Geometry: final body of the model. Coordinates: model frame, mm. Face numbers are marked on the shaded views. A direction names the side the tool comes from. Coordinates: 2 decimals unless noted, no trailing zeros. Order: outer loops, then holes, each group sorted by start corner. A loop starts at its lowest first (then second) coordinate and runs counter-clockwise, first axis right, second up. Notation, with made-up numbers: M 18.25,-35.75 L 35.25,-35.75 A15 ccw 35.25,-9.75 Z; hole C 79,-8 d7. An arc over 180 degrees is marked long. Use CSV: the item, a comma, the result in double quotes. Start each with the question number.
Q1. Mould query, pull axis Y, two halves, no side actions, for the marked faces 1, 2 and 3. Classes: +Y half, -Y half, draft (parallel to the pull), parting line (faces both ways), or undercut.
Q2. Section query C-C, the plane x = 0. Output: boundary loops of the cut face in (y, z).
Q3. Section query B-B, the plane y = 0. Output: boundary loops of the cut face in (x, z), and give its area (3 significant figures).
Q4. Section query A-A, the plane x = 8. Output: boundary loops of the cut face in (y, z), and give its area (3 significant figures).
Q5. Ray query, probe 1 along Y at (x, z) = (8, 1.35); probe 2 along Y at (x, z) = (4.5, 6.75); probe 3 along X at (y, z) = (0.25, 2). Return the intervals inside material, ascending.
Q6. Section query D-D, the plane z = 11.5. Output: boundary loops of the cut face in (x, y).
Q7. Access query for the marked faces 4, 5, 6, 7 and 8. Directions: +Z, -Z, +X, -X, +Y, -Y. A direction counts if a zero-diameter tool reaches every point of the face in a straight line with its end or side. Return the directions, or none.
Q8. First-contact query: P1, Ø6, axis at y = 3, z = 6.5, coming from the -X side; P2, Ø2, axis at x = -0.5, y = -1, coming from the -Z side; P3, Ø4, axis at x = -2.5, y = 0, coming from the +Z side; P4, Ø1.5, axis at y = 6.5, z = 6.5, coming from the +X side. Flat tips, straight axial feed; report the tip coordinate or a pass-through.
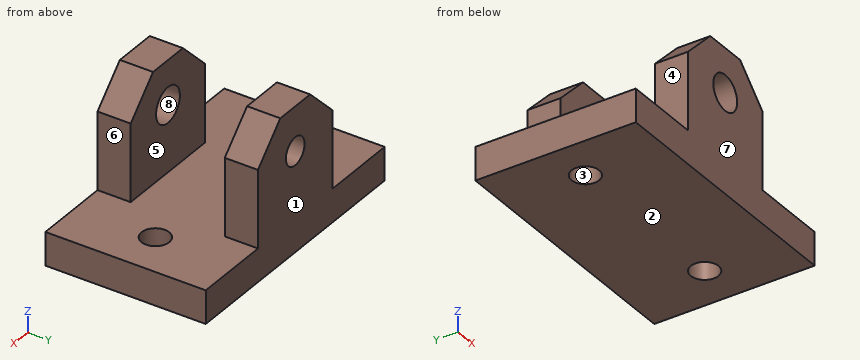
from build123d import *

# Parameters (mm, degrees)
SKETCH_1_W          = 24
SKETCH_1_H          = 14.5
EXTRUDE_1_DEPTH     = 3
SKETCH_2_W          = 10
SKETCH_2_H          = 14
EXTRUDE_1_2_DEPTH   = 3
CUT_EXTRUDE_1_REACH = 25.457
SKETCH_3_R          = 1.6
HOLE_WIZARD_M3_2_D  = 2.5
HOLE_WIZARD_M3_1_D  = 2.5
SKETCH_10_W         = 0.5
SKETCH_10_H         = 14.5
CUT_EXTRUDE_2_DEPTH = 20.813190051
SKETCH_11_W         = 10
SKETCH_11_H         = 1
CUT_EXTRUDE_3_DEPTH = 24.205602772
CHAMFER_1_SIZE      = 3
SKETCH_12_W         = 0.5
SKETCH_12_H         = 14.5
EXTRUDE_2_DEPTH     = 3


with BuildPart() as part:
    # 草图1 → Extrude 1 (new body)
    with BuildSketch(Plane.XY):
        Rectangle(SKETCH_1_W, SKETCH_1_H)
    extrude(amount=EXTRUDE_1_DEPTH)

    # 草图2 → Extrude 1 2 (add)
    with BuildSketch(Plane.XZ.offset(7.25)):
        with Locations((0, 7)):
            Rectangle(SKETCH_2_W, SKETCH_2_H)
    extrude_1_2 = extrude(amount=-EXTRUDE_1_2_DEPTH)

    # 镜向1: Extrude 1 2 across plane
    add(extrude_1_2.mirror(Plane.ZX))

    # 草图3 → 切除-拉伸1 (cut, up to next)
    with BuildSketch(Plane.XZ.offset(7.25), mode=Mode.PRIVATE) as cut_extrude_1_sk1:
        with Locations(Location((0, 9, 0), (0, 0, 270))):
            Circle(SKETCH_3_R)
    cut_extrude_1_tool1 = extrude(cut_extrude_1_sk1.sketch, amount=-CUT_EXTRUDE_1_REACH, mode=Mode.PRIVATE) & part.part
    add(cut_extrude_1_tool1.solids().sort_by_distance((0, -7.25, 9))[0], mode=Mode.SUBTRACT)

    # M3 螺纹孔2 (through all)
    with Locations(Plane(origin=(0, 7.25, 9), x_dir=(0, 0, 1), z_dir=(0, 1, 0))):
        with Locations((0, 0)):
            Hole(HOLE_WIZARD_M3_2_D / 2)

    # M3 螺纹孔1 (through all)
    with Locations(Plane.XY.offset(3)):
        with Locations((-8, 0), (8, 0)):
            Hole(HOLE_WIZARD_M3_1_D / 2)

    # 草图10 → 切除-拉伸2 (cut, through all)
    with BuildSketch(Plane(origin=(0, 0, 0), x_dir=(-1, 0, 0), z_dir=(0, 0, -1))):
        with Locations((-11.75, 0)):
            Rectangle(SKETCH_10_W, SKETCH_10_H)
        with Locations((11.75, 0)):
            Rectangle(SKETCH_10_W, SKETCH_10_H)
    extrude(amount=-CUT_EXTRUDE_2_DEPTH, mode=Mode.SUBTRACT)

    # 草图11 → 切除-拉伸3 (cut, through all)
    with BuildSketch(Plane.XZ.offset(7.25)):
        with Locations((0, 13.5)):
            Rectangle(SKETCH_11_W, SKETCH_11_H)
    extrude(amount=-CUT_EXTRUDE_3_DEPTH, mode=Mode.SUBTRACT)

    # 倒角1
    chamfer_1_edges = [part.edges().sort_by_distance(p)[0] for p in [
        (5, -5.75, 13),
        (-5, -5.75, 13),
        (-5, 5.75, 13),
        (5, 5.75, 13),
    ]]
    chamfer(chamfer_1_edges, length=CHAMFER_1_SIZE)

    # 草图12 → 凸台-拉伸2 (add)
    with BuildSketch(Plane.XY.offset(3)):
        with Locations((11.75, 0)):
            Rectangle(SKETCH_12_W, SKETCH_12_H)
    extrude_2 = extrude(amount=-EXTRUDE_2_DEPTH)

    # 镜向2: 凸台-拉伸2 across plane
    add(extrude_2.mirror(Plane(origin=(0, 0, 0), x_dir=(0, 0, 1), z_dir=(1, 0, 0))))


solid = part.part
Responses:
1,face 1,"+Y half"
1,face 2,"draft"
1,face 3,"undercut"
2,outline,"M -7.25,0 L 7.25,0 L 7.25,7.75 L 4.25,7.75 L 4.25,3 L -4.25,3 L -4.25,7.4 L -7.25,7.4 Z; M -7.25,10.6 L -4.25,10.6 L -4.25,13 L -7.25,13 Z; M 4.25,10.25 L 7.25,10.25 L 7.25,13 L 4.25,13 Z"
3,outline,"M -12,0 L -9.25,0 L -9.25,3 L -12,3 Z; M -6.75,0 L 6.75,0 L 6.75,3 L -6.75,3 Z; M 9.25,0 L 12,0 L 12,3 L 9.25,3 Z"
3,area,"57.0 mm²"
4,outline,"M -7.25,0 L -1.25,0 L -1.25,3 L -7.25,3 Z; M 1.25,0 L 7.25,0 L 7.25,3 L 1.25,3 Z"
4,area,"36.0 mm²"
5,probe 1,"y = -7.25 to -1.25, 1.25 to 7.25"
5,probe 2,"y = -7.25 to -4.25, 4.25 to 7.25"
5,probe 3,"x = -12 to -9.22, -6.78 to 6.78, 9.22 to 12"
6,outline,"M -3.5,-7.25 L 3.5,-7.25 L 3.5,-4.25 L -3.5,-4.25 Z; M -3.5,4.25 L 3.5,4.25 L 3.5,7.25 L -3.5,7.25 Z"
7,face 4,"+Z, -X, +Y, -Y"
7,face 5,"+Z, +X, -X"
7,face 6,"+Z, +X, +Y, -Y"
7,face 7,"+Z, -Z, +X, -X, -Y"
7,face 8,"-Y"
8,P1,"stops at x = -5"
8,P2,"stops at z = 0"
8,P3,"stops at z = 3"
8,P4,"stops at x = 5"
